```python
from build123d import *

# Parameters (mm, degrees)
F0_R     = 10
F0_R_2   = 20
F1_DEPTH = 25
F2_DEPTH = 25
F3_DEPTH = 25
F4_DEPTH = 25
F5_DEPTH = 25


with BuildPart() as f1:
    # F0 (on Top) → F1 (new body)
    with BuildSketch(Plane.XY):
        with BuildLine():
            Line((69.319781, 74.291547), (-54.680219, 74.291547))
            Line((-54.680219, 74.291547), (-54.680219, -8.708453))
            Line((-54.680219, -8.708453), (0.319781, -8.708453))
            ThreePointArc((0.319781, -8.708453), (10.926383, -13.101851), (15.319781, -23.708453))
            Line((15.319781, -23.708453), (15.319781, -28.708453))
            Line((15.319781, -28.708453), (69.319781, -28.708453))
            Line((69.319781, -28.708453), (69.319781, 74.291547))
        make_face()
        with Locations((-24.680219, 9.291547)):
            Circle(F0_R, mode=Mode.SUBTRACT)
        with Locations((45.319781, 4.291547)):
            Circle(F0_R_2, mode=Mode.SUBTRACT)
        with BuildLine():
            ThreePointArc((-14.680219, 53.291547), (-12.629966, 58.241294), (-7.680219, 60.291547))
            Line((-7.680219, 60.291547), (57.319781, 60.291547))
            ThreePointArc((57.319781, 60.291547), (62.269529, 58.241294), (64.319781, 53.291547))
            Line((64.319781, 53.291547), (64.319781, 51.291547))
            ThreePointArc((64.319781, 51.291547), (62.269529, 46.341799), (57.319781, 44.291547))
            Line((57.319781, 44.291547), (-7.680219, 44.291547))
            ThreePointArc((-7.680219, 44.291547), (-12.629966, 46.341799), (-14.680219, 51.291547))
            Line((-14.680219, 51.291547), (-14.680219, 53.291547))
        make_face(mode=Mode.SUBTRACT)
    extrude(amount=F1_DEPTH)

    # F0 (on Top) → F2 (join)
    with BuildSketch(Plane.XY):
        with BuildLine():
            Line((69.319781, 74.291547), (-54.680219, 74.291547))
            Line((-54.680219, 74.291547), (-54.680219, -8.708453))
            Line((-54.680219, -8.708453), (0.319781, -8.708453))
            ThreePointArc((0.319781, -8.708453), (10.926383, -13.101851), (15.319781, -23.708453))
            Line((15.319781, -23.708453), (15.319781, -28.708453))
            Line((15.319781, -28.708453), (69.319781, -28.708453))
            Line((69.319781, -28.708453), (69.319781, 74.291547))
        make_face()
        with Locations((-24.680219, 9.291547)):
            Circle(F0_R, mode=Mode.SUBTRACT)
        with Locations((45.319781, 4.291547)):
            Circle(F0_R_2, mode=Mode.SUBTRACT)
        with BuildLine():
            ThreePointArc((-14.680219, 53.291547), (-12.629966, 58.241294), (-7.680219, 60.291547))
            Line((-7.680219, 60.291547), (57.319781, 60.291547))
            ThreePointArc((57.319781, 60.291547), (62.269529, 58.241294), (64.319781, 53.291547))
            Line((64.319781, 53.291547), (64.319781, 51.291547))
            ThreePointArc((64.319781, 51.291547), (62.269529, 46.341799), (57.319781, 44.291547))
            Line((57.319781, 44.291547), (-7.680219, 44.291547))
            ThreePointArc((-7.680219, 44.291547), (-12.629966, 46.341799), (-14.680219, 51.291547))
            Line((-14.680219, 51.291547), (-14.680219, 53.291547))
        make_face(mode=Mode.SUBTRACT)
    extrude(amount=F2_DEPTH)

    # F0 (on Top) → F3 (join)
    with BuildSketch(Plane.XY):
        with BuildLine():
            Line((69.319781, 74.291547), (-54.680219, 74.291547))
            Line((-54.680219, 74.291547), (-54.680219, -8.708453))
            Line((-54.680219, -8.708453), (0.319781, -8.708453))
            ThreePointArc((0.319781, -8.708453), (10.926383, -13.101851), (15.319781, -23.708453))
            Line((15.319781, -23.708453), (15.319781, -28.708453))
            Line((15.319781, -28.708453), (69.319781, -28.708453))
            Line((69.319781, -28.708453), (69.319781, 74.291547))
        make_face()
        with Locations((-24.680219, 9.291547)):
            Circle(F0_R, mode=Mode.SUBTRACT)
        with Locations((45.319781, 4.291547)):
            Circle(F0_R_2, mode=Mode.SUBTRACT)
        with BuildLine():
            ThreePointArc((-14.680219, 53.291547), (-12.629966, 58.241294), (-7.680219, 60.291547))
            Line((-7.680219, 60.291547), (57.319781, 60.291547))
            ThreePointArc((57.319781, 60.291547), (62.269529, 58.241294), (64.319781, 53.291547))
            Line((64.319781, 53.291547), (64.319781, 51.291547))
            ThreePointArc((64.319781, 51.291547), (62.269529, 46.341799), (57.319781, 44.291547))
            Line((57.319781, 44.291547), (-7.680219, 44.291547))
            ThreePointArc((-7.680219, 44.291547), (-12.629966, 46.341799), (-14.680219, 51.291547))
            Line((-14.680219, 51.291547), (-14.680219, 53.291547))
        make_face(mode=Mode.SUBTRACT)
    extrude(amount=F3_DEPTH)

    # F0 (on Top) → F4 (join)
    with BuildSketch(Plane.XY):
        with BuildLine():
            Line((69.319781, 74.291547), (-54.680219, 74.291547))
            Line((-54.680219, 74.291547), (-54.680219, -8.708453))
            Line((-54.680219, -8.708453), (0.319781, -8.708453))
            ThreePointArc((0.319781, -8.708453), (10.926383, -13.101851), (15.319781, -23.708453))
            Line((15.319781, -23.708453), (15.319781, -28.708453))
            Line((15.319781, -28.708453), (69.319781, -28.708453))
            Line((69.319781, -28.708453), (69.319781, 74.291547))
        make_face()
        with Locations((-24.680219, 9.291547)):
            Circle(F0_R, mode=Mode.SUBTRACT)
        with Locations((45.319781, 4.291547)):
            Circle(F0_R_2, mode=Mode.SUBTRACT)
        with BuildLine():
            ThreePointArc((-14.680219, 53.291547), (-12.629966, 58.241294), (-7.680219, 60.291547))
            Line((-7.680219, 60.291547), (57.319781, 60.291547))
            ThreePointArc((57.319781, 60.291547), (62.269529, 58.241294), (64.319781, 53.291547))
            Line((64.319781, 53.291547), (64.319781, 51.291547))
            ThreePointArc((64.319781, 51.291547), (62.269529, 46.341799), (57.319781, 44.291547))
            Line((57.319781, 44.291547), (-7.680219, 44.291547))
            ThreePointArc((-7.680219, 44.291547), (-12.629966, 46.341799), (-14.680219, 51.291547))
            Line((-14.680219, 51.291547), (-14.680219, 53.291547))
        make_face(mode=Mode.SUBTRACT)
    extrude(amount=F4_DEPTH)

    # F0 (on Top) → F5 (join)
    with BuildSketch(Plane.XY):
        with BuildLine():
            Line((69.319781, 74.291547), (-54.680219, 74.291547))
            Line((-54.680219, 74.291547), (-54.680219, -8.708453))
            Line((-54.680219, -8.708453), (0.319781, -8.708453))
            ThreePointArc((0.319781, -8.708453), (10.926383, -13.101851), (15.319781, -23.708453))
            Line((15.319781, -23.708453), (15.319781, -28.708453))
            Line((15.319781, -28.708453), (69.319781, -28.708453))
            Line((69.319781, -28.708453), (69.319781, 74.291547))
        make_face()
        with Locations((-24.680219, 9.291547)):
            Circle(F0_R, mode=Mode.SUBTRACT)
        with Locations((45.319781, 4.291547)):
            Circle(F0_R_2, mode=Mode.SUBTRACT)
        with BuildLine():
            ThreePointArc((-14.680219, 53.291547), (-12.629966, 58.241294), (-7.680219, 60.291547))
            Line((-7.680219, 60.291547), (57.319781, 60.291547))
            ThreePointArc((57.319781, 60.291547), (62.269529, 58.241294), (64.319781, 53.291547))
            Line((64.319781, 53.291547), (64.319781, 51.291547))
            ThreePointArc((64.319781, 51.291547), (62.269529, 46.341799), (57.319781, 44.291547))
            Line((57.319781, 44.291547), (-7.680219, 44.291547))
            ThreePointArc((-7.680219, 44.291547), (-12.629966, 46.341799), (-14.680219, 51.291547))
            Line((-14.680219, 51.291547), (-14.680219, 53.291547))
        make_face(mode=Mode.SUBTRACT)
    extrude(amount=F5_DEPTH)


solid = f1.part
```
Can you work these out from the model? Positions are in its coordinate system, mm. A direction names the side the tool comes from. Round coordinates to 2 decimals unless told otherwise and drop trailing zeros. Loops run counter-clockwise (first coordinate to the right, second up) from the corner with the lowest first, then second, coordinate; pieces in that order, holes last. Notation, with made-up numbers: (35.5, -34) -> (79.5, -34) arc R27 ccw to (79.5, -6) -> close; hole circle Ø6 at (6, 73). An arc over 180 degrees is marked (long way). Answer in a Markdown table with one row per item.
Item 1: We'd pull the mould along X, two halves only. Please class faces 1 (the cylindrical face through (10.809, -12.986, 12.325)), 2 (the flat face through (24, 60.292, 12)), 3 (the flat face through (42, -28.708, 12)): released by +X, released by -X, zero draft, split by the parting line, or undercut.
Answer block:
| item | result |
|---|---|
| face 1 | released by -X |
| face 2 | undercut |
| face 3 | zero draft |
Item 2: Suppose I cut it at A-A, the plane x = -3.5. List the corners of the cut face in (y, z) for me, plus the area to 4 significant figures.
Answer block:
| item | result |
|---|---|
| outline | (-8.71, 0) -> (44.29, 0) -> (44.29, 25) -> (-8.71, 25) -> close; (60.29, 0) -> (74.29, 0) -> (74.29, 25) -> (60.29, 25) -> close |
| area | 1,675 mm² |
Item 3: Will these pins go through, and if not, where does the flat tip stop? P1, Ø1.5, axis at x = -18.5, z = 15, coming from the -Y side; P2, Ø4, axis at y = -26, z = 10, coming from the -X side.
Answer block:
| item | result |
|---|---|
| P1 | y = -8.71 |
| P2 | x = 15.32 |
Item 4: Suppose I cut it at B-B, the plane y = 12. List the corners of the cut face in (x, z) for me.
Answer block:
| item | result |
|---|---|
| outline | (-54.68, 0) -> (-34.31, 0) -> (-34.31, 25) -> (-54.68, 25) -> close; (-15.05, 0) -> (26.86, 0) -> (26.86, 25) -> (-15.05, 25) -> close; (63.77, 0) -> (69.32, 0) -> (69.32, 25) -> (63.77, 25) -> close |
Item 5: Suppose I cut it at C-C, the plane x = 56. List the corners of the cut face in (y, z) for me.
Answer block:
| item | result |
|---|---|
| outline | (-28.71, 0) -> (-12.62, 0) -> (-12.62, 25) -> (-28.71, 25) -> close; (21.2, 0) -> (44.29, 0) -> (44.29, 25) -> (21.2, 25) -> close; (60.29, 0) -> (74.29, 0) -> (74.29, 25) -> (60.29, 25) -> close |
Item 6: If I drill on probe 1 along X at (y, z) = (51.5, 21.75); probe 2 along Y at (x, z) = (16.5, 11.25); probe 3 along X at (y, z) = (11, 9), over which ranges is the centre line in solid material (lowest first)?
Answer block:
| item | result |
|---|---|
| probe 1 | -54.68 to -14.68, 64.32 to 69.32 |
| probe 2 | -28.71 to 44.29, 60.29 to 74.29 |
| probe 3 | -54.68 to -34.53, -14.83 to 26.48, 64.16 to 69.32 |
Item 7: Suppose I cut it at D-D, the plane z = 20. List the corners of the cut face in (x, y) for me.
Answer block:
| item | result |
|---|---|
| outline | (-54.68, -8.71) -> (0.32, -8.71) arc R15 cw to (15.32, -23.71) -> (15.32, -28.71) -> (69.32, -28.71) -> (69.32, 74.29) -> (-54.68, 74.29) -> close; hole circle Ø20 at (-24.68, 9.29); hole (-14.68, 51.29) arc R7 ccw to (-7.68, 44.29) -> (57.32, 44.29) arc R7 ccw to (64.32, 51.29) -> (64.32, 53.29) arc R7 ccw to (57.32, 60.29) -> (-7.68, 60.29) arc R7 ccw to (-14.68, 53.29) -> close; hole circle Ø40 at (45.32, 4.29) |
Item 8: On a 3-axis mill with a long thin cutter (end or side, diameter ignored), from which of +Z, -Z, +X, -X, +Y, -Y can I reach the whole of each face in a straight line? I mean faces 4 (the cylindrical face through (62.324, 46.397, 12.325)), 5 (the flat face through (15.32, -26, 12)), 6 (the flat face through (69.32, 22, 12)). Say none if no direction works.
Answer block:
| item | result |
|---|---|
| face 4 | +Z, -Z |
| face 5 | +Z, -Z, -X, -Y |
| face 6 | +Z, -Z, +X, +Y, -Y |
